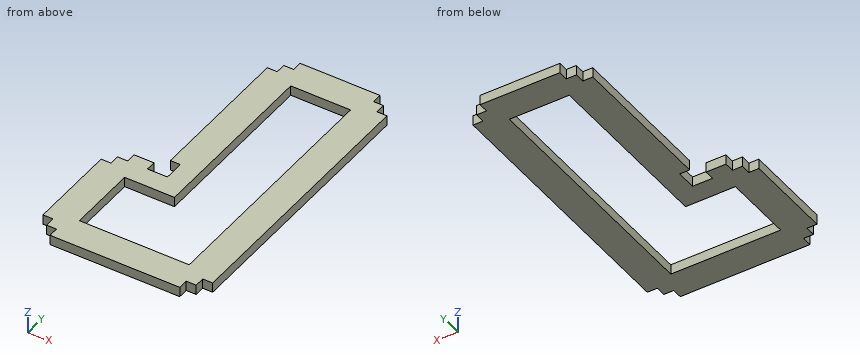
from build123d import *

# Parameters (mm, degrees)
BOSS_EXTRUDE1_START = -3.175
BOSS_EXTRUDE1_DEPTH = 6.35
CUT_EXTRUDE1_DEPTH  = 167.316670842


with BuildPart() as part:
    # Sketch1 → Boss-Extrude1 (new body)
    with BuildSketch(Plane.XY.offset(BOSS_EXTRUDE1_START)):
        Polygon((12.7, -69.85), (19.05, -69.85), (19.05, -76.2), (101.6, -76.2), (101.6, -69.85), (107.95, -69.85), (107.95, -63.5), (114.3, -63.5), (114.3, 107.95), (107.95, 107.95), (107.95, 114.3), (101.6, 114.3), (101.6, 120.65), (50.8, 120.65), (50.8, 114.3), (44.45, 114.3), (44.45, 107.95), (38.1, 107.95), (38.1, 12.7), (44.45, 12.7), (44.45, 0), (31.75, 0), (31.75, 6.35), (19.05, 6.35), (19.05, 0), (12.7, 0), (12.7, -6.35), (6.35, -6.35), (6.35, -63.5), (12.7, -63.5), align=None)
    extrude(amount=-BOSS_EXTRUDE1_DEPTH)

    # Sketch2 → Cut-Extrude1 (cut, through all)
    with BuildSketch(Plane.XY.offset(-3.175)):
        Polygon((25.4, -57.15), (95.25, -57.15), (95.25, 101.6), (57.15, 101.6), (57.15, -12.7), (25.4, -12.7), align=None)
    extrude(amount=-CUT_EXTRUDE1_DEPTH, mode=Mode.SUBTRACT)


solid = part.part
Could you check a few things on this model? Use its own coordinates, in mm. Round coordinates to 2 decimals unless told otherwise and drop trailing zeros. Order: outer loops, then holes, each group sorted by start corner. A loop starts at its lowest first (then second) coordinate and runs counter-clockwise, first axis right, second up.
(1) Imagine slicing it at C-C (y = 4.5). Write out the boundary of the cut face in (x, z) (3 decimals).
Response values:
outline: (19.05, -9.525) - (31.75, -9.525) - (31.75, -3.175) - (19.05, -3.175) - close; (44.45, -9.525) - (57.15, -9.525) - (57.15, -3.175) - (44.45, -3.175) - close; (95.25, -9.525) - (114.3, -9.525) - (114.3, -3.175) - (95.25, -3.175) - close
(2) Imagine slicing it at B-B (y = 72). Write out the boundary of the cut face in (x, z) (3 decimals), plus the area to 3 significant figures.
Response values:
outline: (38.1, -9.525) - (57.15, -9.525) - (57.15, -3.175) - (38.1, -3.175) - close; (95.25, -9.525) - (114.3, -9.525) - (114.3, -3.175) - (95.25, -3.175) - close
area: 242 mm2
(3) I'm going to push flat-ended pins straight in: pin 1 (3 mm diameter, centred on x = 104, z = -6.5, fed in from +Y); pin 2 (1.9 mm diameter, centred on x = 15, z = -7, fed in from +Y); pin 3 (1.9 mm diameter, centred on y = 117.5, z = -6, fed in from -X). Where does each tip first touch, or does it pass through?
Response values:
pin 1: stops at y = 114.3
pin 2: stops at y = 0
pin 3: stops at x = 50.8
(4) Please list where these lines run through material, in increasing order: line 1 along Y through (x, z) = (71.5, -8.75); line 2 along Y through (x, z) = (31, -7.5); line 3 along X through (y, z) = (8, -6.25).
Response values:
line 1: y = -76.2 to -57.15, 101.6 to 120.65
line 2: y = -76.2 to -57.15, -12.7 to 6.35
line 3: x = 44.45 to 57.15, 95.25 to 114.3
(5) Imagine slicing it at A-A (x = 86.5). Write out the boundary of the cut face in (y, z) (3 decimals).
Response values:
outline: (-76.2, -9.525) - (-57.15, -9.525) - (-57.15, -3.175) - (-76.2, -3.175) - close; (101.6, -9.525) - (120.65, -9.525) - (120.65, -3.175) - (101.6, -3.175) - close
